```python
from build123d import *

# Parameters (mm, degrees)
F1_DEPTH       = 63.5
F2_DEPTH       = 25.4
F3_DEPTH       = 7.9375
F5_R           = 6.35
F7_D           = 5
F7_CSINK_D     = 10
F7_CSINK_ANGLE = 90


# Not quite as in the source:
# - a feature names something its author has since deleted; it is built from what else it names


with BuildPart() as f1:
    # F0 (on Front) → F1 (new body, symmetric)
    with BuildSketch(Plane.XZ):
        Polygon((31.75, 9.525), (-50.8, 9.525), (-50.8, -9.525), (50.8, -9.525), (50.8, 9.525), align=None)
    extrude(amount=F1_DEPTH, both=True)

    # F0 (on Front) → F2 (join, symmetric)
    with BuildSketch(Plane.XZ):
        with BuildLine():
            Line((31.75, 27.0002), (31.75, 9.525))
            Line((31.75, 9.525), (50.8, 9.525))
            Line((50.8, 9.525), (50.8, 27.0002))
            ThreePointArc((50.8, 27.0002), (55.4496798487, 38.2255201513), (66.675, 42.8752))
            Line((66.675, 42.8752), (69.85, 42.8752))
            Line((69.85, 42.8752), (69.85, 61.9252))
            Line((69.85, 61.9252), (66.675, 61.9252))
            add(Edge.make_bspline(
                [(65.9455207974, 61.9175808453), (66.1893918553, 61.9205374951), (66.4325563897, 61.9230769491), (66.675, 61.9252)],
                knots=[127.9589342237, 127.9589342237, 127.9589342237, 127.9589342237, 128.6318645789, 128.6318645789, 128.6318645789, 128.6318645789], degree=3))
            ThreePointArc((65.9455207974, 61.9175808453), (41.72271868, 51.4366334944), (31.75, 27.0002))
        make_face()
        Polygon((69.85, 66.675), (69.85, 61.9252), (69.85, 42.8752), (95.25, 42.8752), (95.25, 66.675), align=None)
    extrude(amount=F2_DEPTH, both=True)

    # F0 (on Front) → F3 (join, symmetric)
    with BuildSketch(Plane.XZ):
        with BuildLine():
            add(Edge.make_bspline(
                [(-50.8, 9.525), (-52.3458055459, 45.7083043223), (19.5729944142, 61.3553684788), (65.9455207974, 61.9175808453)],
                knots=[0, 0, 0, 0, 127.9589342237, 127.9589342237, 127.9589342237, 127.9589342237], degree=3))
            Line((-50.8, 9.525), (31.75, 9.525))
            Line((31.75, 9.525), (31.75, 27.0002))
            ThreePointArc((31.75, 27.0002), (41.72271868, 51.4366334944), (65.9455207974, 61.9175808453))
        make_face()
    extrude(amount=F3_DEPTH, both=True)

    # F0 (on Front) → F4 (revolve)
    with BuildSketch(Plane.XZ):
        Polygon((120.65, 66.675), (95.25, 66.675), (95.25, 42.8752), (95.25, 38.1), (120.65, 38.1), align=None)
    revolve(axis=Axis((95.25, 0, 52.3875), (0, 0, 1)))

    # F5
    f5_edges = [f1.edges().sort_by_distance(p)[0] for p in [
        (50.8, -63.5, 0),
        (-50.8, -63.5, 0),
        (-50.8, 63.5, 0),
        (50.8, 63.5, 0),
    ]]
    fillet(f5_edges, radius=F5_R)

    # F7 (through all)
    with Locations(Plane.XY.offset(9.525)):
        with Locations((0, 36.2676680088), (0, -38.4938158095)):
            CounterSinkHole(F7_D / 2, F7_CSINK_D / 2, counter_sink_angle=F7_CSINK_ANGLE)


solid = f1.part
```
Input: part model. Units: mm. Frame: model coordinates. A direction names the side the tool comes from. Coordinates: 2 decimals unless noted, no trailing zeros. Write each loop counter-clockwise with the first axis right and the second up, starting at its lowest first coordinate (ties: lowest second). Pieces come first, ordered by that corner, then holes. Notation, with made-up numbers: M -27.5,52 L 4.5,52 A11 cw 4.5,57 Z; hole C 64,-30.75 d7. An arc over 180 degrees is marked long. Use one line per item in the form item = value.
Q1. Material intervals for probe 1 along Y at (x, z) = (0, -3.5); probe 2 along Z at (x, y) = (73, 1) (3 decimals); probe 3 along X at (y, z) = (8, 3), sorted ascending. Write a range as from..to.
Answer below:
probe_1 = -63.5..-40.99, -35.99..33.77, 38.77..63.5
probe_2 = 38.1..66.675
probe_3 = -50.8..50.8
Q2. Set-up query: faces 1 (the face through (-6, 7.938, 30)), 2 (the face through (50.8, -1, 4)), 3 (the face through (63, 25.4, 45)), 4 (the face through (31.75, -17, 18)), 5 (the face through (63, -25.4, 45)). Return all of +Z, -Z, +X, -X, +Y, -Y with unobstructed straight access to the full face (end or side cutting, diameter ignored); none if empty.
Answer below:
face_1 = +Z, -X, +Y
face_2 = -Z, +X, +Y, -Y
face_3 = +Z, +X, -X, +Y
face_4 = +Z, -X, -Y
face_5 = +Z, +X, -X, -Y
Q3. Draft query along X for faces 6 (the face through (1, 42, 9.525)), 7 (the face through (-50.8, -1, 0)), 8 (the face through (48.89, -61.69, 0.13)), 9 (the face through (69, 2, 42.875)). Return one class per face: released by +X, released by -X, zero draft, split by the parting line, or undercut.
Answer below:
face_6 = zero draft
face_7 = released by -X
face_8 = released by +X
face_9 = undercut
Q4. First-contact query: pin 1 (1 mm diameter, centred on x = 67.5, y = -1, fed in from +Z); pin 2 (6 mm diameter, centred on x = 94, z = 37.5, fed in from +Y); pin 3 (21 mm diameter, centred on y = 25.5, z = 0, fed in from -X). Flat tips, straight axial feed; report the tip coordinate or a pass-through.
Answer below:
pin_1 = 61.93
pin_2 = 25.4
pin_3 = -50.8
Q5. Section B-B (x = 109.5). Return loops of the section in (y, z) (3 decimals), plus the area to 3 significant figures.
Answer below:
outline = M -21.026,38.1 L 21.026,38.1 L 21.026,66.675 L -21.026,66.675 Z
area = 1,200 mm²
Q6. Section A-A (x = 0). Count the separate pieces of the cut face and the enclosed holes in it, plus the area to 3 significant figures.
Answer below:
separate_pieces = 3
enclosed_holes = 0
area = 2,900 mm²
